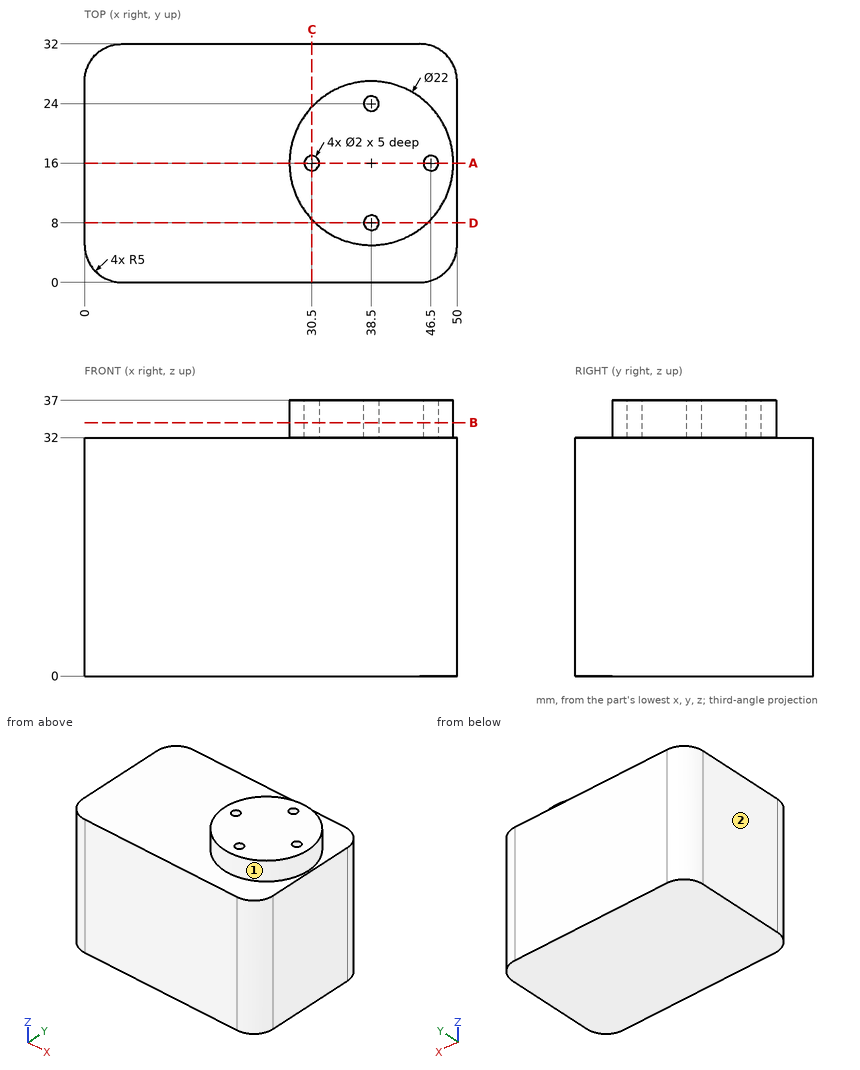
Design review of the part shown in the three views and the two pictorial views. Dimensions are in mm from the part's minimum x, y and z. A direction names the side the tool comes from. Give positions to 0.01 mm unless a question says otherwise; leave off trailing zeros. Write each loop counter-clockwise with the first axis right and the second up, starting at its lowest first coordinate (ties: lowest second). Pieces come first, ordered by that corner, then holes. Notation, with made-up numbers: (20.5, -2.5) -> (65.5, -2.5) arc R17 cw to (65.5, 4.5) -> close; hole circle Ø10 at (3.5, -26.5). An arc over 180 degrees is marked (long way). Answer in a Markdown table with one row per item.
1) Clearance check with flat-ended pins moving along their axes: P1, Ø2, axis at x = 46, y = 16.5, coming from the +Z side; P2, Ø4, axis at x = 13.5, y = 25, coming from the +Z side. State where each tip first meets the part, or that it passes through.
Worked answers:
| item | result |
|---|---|
| P1 | z = 37 |
| P2 | z = 32 |
2) Add section B-B on z = 34. State the section outline as (x, y) points, plus the area to 3 significant figures.
Worked answers:
| item | result |
|---|---|
| outline | circle Ø22 at (38.5, 16); hole circle Ø2 at (30.5, 16); hole circle Ø2 at (38.5, 8); hole circle Ø2 at (38.5, 24); hole circle Ø2 at (46.5, 16) |
| area | 368 mm² |
3) Add section A-A on y = 16. State the section outline as (x, z) points, plus the area to 3 significant figures.
Worked answers:
| item | result |
|---|---|
| outline | (0, 0) -> (50, 0) -> (50, 32) -> (49.5, 32) -> (49.5, 37) -> (47.5, 37) -> (47.5, 32) -> (45.5, 32) -> (45.5, 37) -> (31.5, 37) -> (31.5, 32) -> (29.5, 32) -> (29.5, 37) -> (27.5, 37) -> (27.5, 32) -> (0, 32) -> close |
| area | 1,690 mm² |
4) Add section D-D on y = 8. State the section outline as (x, z) points.
Worked answers:
| item | result |
|---|---|
| outline | (0, 0) -> (50, 0) -> (50, 32) -> (46.05, 32) -> (46.05, 37) -> (39.5, 37) -> (39.5, 32) -> (37.5, 32) -> (37.5, 37) -> (30.95, 37) -> (30.95, 32) -> (0, 32) -> close |
5) Tool access review of the marked faces 1 and 2: name each direction out of +Z, -Z, +X, -X, +Y, -Y from which nothing blocks a thin tool from reaching the whole face with its end or side.
Worked answers:
| item | result |
|---|---|
| face 1 | +Z |
| face 2 | +Z, -Z, -X, +Y, -Y |
6) For L1, parallel to Y at x = 38, z = 34; L2, parallel to Z at x = 18, y = 16; L3, parallel to Y at x = 46.5, z = 35.1, list the stretches that pass through material, from the lowest coordinate up. Write a range as [from, to].
Worked answers:
| item | result |
|---|---|
| L1 | [5.01, 7.13], [8.87, 23.13], [24.87, 26.99] |
| L2 | [0, 32] |
| L3 | [8.45, 15], [17, 23.55] |
7) Add section C-C on x = 30.5. State the section outline as (y, z) points, plus the area to 3 significant figures.
Worked answers:
| item | result |
|---|---|
| outline | (0, 0) -> (32, 0) -> (32, 32) -> (23.55, 32) -> (23.55, 37) -> (17, 37) -> (17, 32) -> (15, 32) -> (15, 37) -> (8.45, 37) -> (8.45, 32) -> (0, 32) -> close |
| area | 1,090 mm² |
